The model under review builds one solid part; all positions refer to its coordinate system, in mm. Face numbers are marked on the shaded views. A direction names the side the tool comes from. Coordinates: 2 decimals unless noted, no trailing zeros. Write each loop counter-clockwise with the first axis right and the second up, starting at its lowest first coordinate (ties: lowest second). Pieces come first, ordered by that corner, then holes.
1) Add section A-A, the plane x = 0. State the section outline as (y, z) points, then the cut area to 3 significant figures.
2) Machinability: for the marked faces 1 and 2, which of the approach directions +Z, -Z, +X, -X, +Y, -Y give a long, thin tool a straight path to every point of the face, cutting with its end or side? Answer none if there is none.
3) For line 1 (Y direction, x = 0, z = 42); line 2 (Y direction, x = 5, z = -38.5) (3 decimals); line 3 (Z direction, x = 4, y = -16.5), list the stretches that pass through material, from the lowest coordinate up.
4) Add section D-D, the plane z = -16. State the section outline as (x, y) points.
5) For P1, Ø5, axis at x = 3, y = -1, coming from the +Z side; P2, Ø8, axis at x = -19.5, y = -30.5, coming from the -Z side; P3, Ø3, axis at x = -30.5, z = -1, coming from the -Y side, all flat-tipped, find the tip position at first contact; note any pin that passes through.
6) Mouldability with a two-part tool opening along Y and no side actions: class the marked faces 3, 4 and 5 as released by +Y, released by -Y, zero draft, split by the parting line, or undercut.
7) Add section C-C, the plane z = -44. State the section outline as (x, y) points.
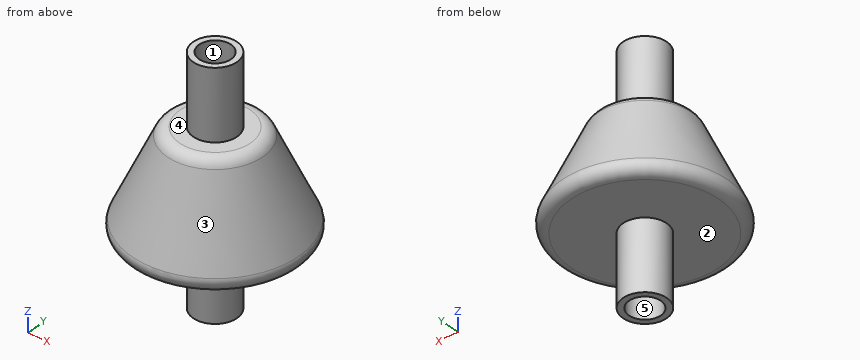
from build123d import *

# Parameters (mm, degrees)
SKETCH1_R           = 11
SKETCH1_R_2         = 8
BOSS_EXTRUDE1_DEPTH = 60


with BuildPart() as part:
    # Sketch1 → Boss-Extrude1 (new, symmetric)
    with BuildSketch(Plane.XY):
        Circle(SKETCH1_R)
        Circle(SKETCH1_R_2, mode=Mode.SUBTRACT)
    extrude(amount=BOSS_EXTRUDE1_DEPTH, both=True)

    # Sketch2 → Revolve1 (revolve)
    with BuildSketch(Plane(origin=(0, 0, 0), x_dir=(0, 0, -1), z_dir=(1, 0, 0)), mode=Mode.PRIVATE) as revolve1_sk:
        with BuildLine():
            Line((-25, 0), (-25, 17.840263865))
            ThreePointArc((-25, 17.840263865), (-23.93794832, 21.458657097), (-21.088750877, 23.929041134))
            Line((-21.088750877, 23.929041134), (17.921053029, 41.76363109))
            ThreePointArc((17.921053029, 41.76363109), (22.702338353, 41.423150362), (25, 37.21632645))
            Line((25, 37.21632645), (25, 0))
            Line((25, 0), (-25, 0))
        make_face()
    revolve(revolve1_sk.sketch.rotate(Axis((0, 0, -25), (0, 0, 1)), 90), axis=Axis((0, 0, -25), (0, 0, 1)))


solid = part.part
Geometry results:
1. outline: (-41.76, -17.92) arc R5 ccw to (-37.22, -25) - (-11, -25) - (-11, -60) - (-8, -60) - (-8, -25) - (8, -25) - (8, -60) - (11, -60) - (11, -25) - (37.22, -25) arc R5 ccw to (41.76, -17.92) - (23.93, 21.09) arc R6.69 ccw to (17.84, 25) - (11, 25) - (11, 60) - (8, 60) - (8, 25) - (-8, 25) - (-8, 60) - (-11, 60) - (-11, 25) - (-17.84, 25) arc R6.69 ccw to (-23.93, 21.09) - close
1. area: 3,740 mm2
2. face 1: +Z
2. face 2: -Z
3. line 1: y = -11 to -8, 8 to 11
3. line 2: y = -9.798 to -6.245, 6.245 to 9.798
3. line 3: z = -25 to 25
4. outline: circle Ø81.77 at (0, 0)
5. P1: stops at z = 25
5. P2: stops at z = -25
5. P3: stops at y = -18.13
6. face 3: split by the parting line
6. face 4: zero draft
6. face 5: undercut
7. outline: circle Ø22 at (0, 0); hole circle Ø16 at (0, 0)
